from build123d import *

# Parameters (mm, degrees)
SKETCH2_W                    = 82.55
SKETCH2_H                    = 12.7
F_10_0_1935_DIAMETER_HOLE1_D = 4.9149
CIRPATTERN3_COUNT            = 3
CUT_EXTRUDE1_DEPTH           = 13.7
FILLET1_R                    = 4
CIRPATTERN4_COUNT            = 6
FILLET1_OF_CIRPATTERN4_R     = 4
CHAMFER2_SIZE                = 1
F_3_8_0_375_DIAMETER_HOLE1_D = 9.525


with BuildPart() as part:
    # Sketch2 → Revolve1 (revolve)
    with BuildSketch(Plane(origin=(0, 0, 0), x_dir=(0, 0, -1), z_dir=(1, 0, 0))):
        with Locations((-41.275, 6.35)):
            Rectangle(SKETCH2_W, SKETCH2_H)
    revolve(axis=Axis((0, -0.635, 0), (0, 1, 0)))

    # #10 (0.1935) Diameter Hole1 (through all)
    with Locations(Plane(origin=(0, 12.7, 0), x_dir=(1, 0, 0), z_dir=(0, 1, 0))):
        with Locations((-35, 60.621778)):
            f_10_0_1935_diameter_hole1 = Hole(F_10_0_1935_DIAMETER_HOLE1_D / 2)

    # CirPattern3: #10 (0.1935) Diameter Hole1 ×3 about axis
    cirpattern3_axis = Axis((0, 0, 0), (0, 1, 0))
    for i in range(1, CIRPATTERN3_COUNT):
        add(f_10_0_1935_diameter_hole1.rotate(cirpattern3_axis, i * 360 / CIRPATTERN3_COUNT), mode=Mode.SUBTRACT)

    # Sketch8 → Cut-Extrude1 (cut, through all)
    with BuildSketch(Plane(origin=(0, 12.7, 0), x_dir=(1, 0, 0), z_dir=(0, 1, 0))):
        with BuildLine():
            Line((-7.917322, 23.713203), (-34.364196, 69.520533))
            ThreePointArc((-34.364196, 69.520533), (0, 77.55), (34.364196, 69.520533))
            Line((34.364196, 69.520533), (7.917322, 23.713203))
            ThreePointArc((7.917322, 23.713203), (0, 25), (-7.917322, 23.713203))
        make_face()
    cut_extrude1 = extrude(amount=-CUT_EXTRUDE1_DEPTH, mode=Mode.SUBTRACT)

    # Fillet1
    fillet1_edges = [part.edges().sort_by_distance(p)[0] for p in [
        (7.917322, 6.35, -23.713203),
        (-7.917322, 6.35, -23.713203),
        (-34.364196, 6.35, -69.520533),
        (34.364196, 6.35, -69.520533),
    ]]
    fillet(fillet1_edges, radius=FILLET1_R)

    # CirPattern4: Cut-Extrude1 ×6 about axis
    cirpattern4_axis = Axis((0, 0, 0), (0, 1, 0))
    for i in range(1, CIRPATTERN4_COUNT):
        add(cut_extrude1.rotate(cirpattern4_axis, i * 360 / CIRPATTERN4_COUNT), mode=Mode.SUBTRACT)

    # Fillet1 of CirPattern4
    fillet1_of_cirpattern4_edges = [part.edges().sort_by_distance(p)[0] for p in [
        (-16.577576, 6.35, -18.713203),
        (-24.494897, 6.35, -5),
        (-77.388646, 6.35, -5),
        (-43.02445, 6.35, -64.520533),
        (-24.494897, 6.35, 5),
        (-16.577576, 6.35, 18.713203),
        (-43.02445, 6.35, 64.520533),
        (-77.388646, 6.35, 5),
        (-7.917322, 6.35, 23.713203),
        (7.917322, 6.35, 23.713203),
        (34.364196, 6.35, 69.520533),
        (-34.364196, 6.35, 69.520533),
        (16.577576, 6.35, 18.713203),
        (24.494897, 6.35, 5),
        (77.388646, 6.35, 5),
        (43.02445, 6.35, 64.520533),
        (24.494897, 6.35, -5),
        (16.577576, 6.35, -18.713203),
        (43.02445, 6.35, -64.520533),
        (77.388646, 6.35, -5),
    ]]
    fillet(fillet1_of_cirpattern4_edges, radius=FILLET1_OF_CIRPATTERN4_R)

    # Chamfer2
    chamfer2_edges = [part.edges().sort_by_distance(p)[0] for p in [
        (0, 0, -82.55),
    ]]
    chamfer(chamfer2_edges, length=CHAMFER2_SIZE)

    # 3/8 (0.375) Diameter Hole1 (through all)
    with Locations(Plane(origin=(0, 0, 0), x_dir=(-1, 0, 0), z_dir=(0, -1, 0))):
        with Locations((0, 0)):
            Hole(F_3_8_0_375_DIAMETER_HOLE1_D / 2)


solid = part.part
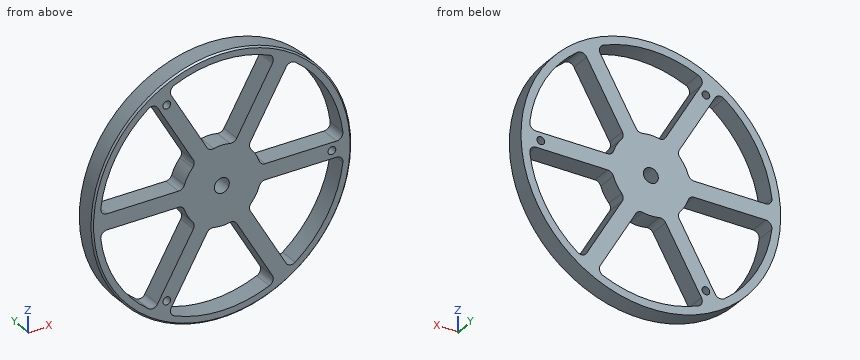
Model file for the job. Use its own axes, mm. Round coordinates to 2 decimals unless told otherwise and drop trailing zeros. Loops run counter-clockwise (first coordinate to the right, second up) from the corner with the lowest first, then second, coordinate; pieces in that order, holes last.
1. Band-saw the part on C-C, the plane x = 36.5. Count the separate pieces of the cut face and the enclosed holes in it, and give its area (3 significant figures).
Check values:
separate pieces: 3
enclosed holes: 0
area: 655 mm2
2. Drop flat-ended pins along their axis: P1, Ø4, axis at x = -35, z = 60.62, coming from the -Y side; P2, Ø1, axis at x = 46, y = 7, coming from the -Z side; P3, Ø4, axis at x = 56, y = 8, coming from the +Z side; P4, Ø3, axis at y = 1.5, z = 47.5, coming from the +X side. Give the stop position or say it passes through.
Check values:
P1: passes through
P2: stops at z = -68.88
P3: stops at z = 62.44
P4: stops at x = 68.55
3. Band-saw the part on A-A, the plane z = 0. List the corners of the cut face in (x, y), and give its area (3 significant figures).
Check values:
outline: (-82.55, 1) - (-81.55, 0) - (-4.76, 0) - (-4.76, 12.7) - (-82.55, 12.7) - close; (4.76, 0) - (67.54, 0) - (67.54, 12.7) - (4.76, 12.7) - close; (72.46, 0) - (81.55, 0) - (82.55, 1) - (82.55, 12.7) - (72.46, 12.7) - close
area: 1,910 mm2
4. Band-saw the part on B-B, the plane x = 0. List the corners of the cut face in (y, z).
Check values:
outline: (0, -81.55) - (1, -82.55) - (12.7, -82.55) - (12.7, -77.55) - (0, -77.55) - close; (0, -25) - (12.7, -25) - (12.7, -4.76) - (0, -4.76) - close; (0, 4.76) - (12.7, 4.76) - (12.7, 25) - (0, 25) - close; (0, 77.55) - (12.7, 77.55) - (12.7, 82.55) - (1, 82.55) - (0, 81.55) - close
5. Wall check: probe 1 along X at (y, z) = (9.5, -22.5); probe 2 along Z at (x, y) = (-35, 8.5); probe 3 along Z at (x, y) = (4, 11). Give the ranges that are in metal, low to high.
Check values:
probe 1: x = -79.42 to -74.21, -18.76 to 18.76, 74.21 to 79.42
probe 2: z = -74.76 to -63.08, -58.16 to -50.62, -5 to 5, 50.62 to 58.16, 63.08 to 74.76
probe 3: z = -82.45 to -77.45, -24.68 to -2.58, 2.58 to 24.68, 77.45 to 82.45
